```python
from build123d import *

# Parameters (mm, degrees)
BOSS_EXTRUDE1_DEPTH = 31.75
SKETCH2_R           = 1.366728635
CUT_EXTRUDE1_DEPTH  = 4.175
SKETCH4_W           = 7.9375
SKETCH4_H           = 4.7625
CUT_EXTRUDE2_DEPTH  = 4.175


with BuildPart() as part:
    # Sketch1 → Boss-Extrude1 (new body)
    with BuildSketch(Plane.XY):
        Polygon((0, 0), (25.4, 0), (25.4, 3.175), (3.175, 3.175), (3.175, 38.1), (0, 38.1), align=None)
    extrude(amount=BOSS_EXTRUDE1_DEPTH)

    # Sketch2 → Cut-Extrude1 (cut, through all)
    with BuildSketch(Plane(origin=(3.175, 0, 0), x_dir=(0, 0, -1), z_dir=(1, 0, 0))):
        with Locations((-25.4, 28.575)):
            Circle(SKETCH2_R)
        with Locations((-6.35, 28.575)):
            Circle(SKETCH2_R)
        with Locations((-25.4, 9.525)):
            Circle(SKETCH2_R)
        with Locations((-6.35, 9.525)):
            Circle(SKETCH2_R)
    extrude(amount=-CUT_EXTRUDE1_DEPTH, mode=Mode.SUBTRACT)

    # Sketch4 → Cut-Extrude2 (cut, through all)
    with BuildSketch(Plane(origin=(0, 3.175, 0), x_dir=(1, 0, 0), z_dir=(0, 1, 0))):
        with Locations((10.31875, -21.43125)):
            Rectangle(SKETCH4_W, SKETCH4_H)
        with Locations((10.31875, -10.31875)):
            Rectangle(SKETCH4_W, SKETCH4_H)
    extrude(amount=-CUT_EXTRUDE2_DEPTH, mode=Mode.SUBTRACT)


solid = part.part
```
Model file for the job. Use its own axes, mm. A direction names the side the tool comes from. Give positions to 0.01 mm unless a question says otherwise; leave off trailing zeros. Loops run counter-clockwise (first coordinate to the right, second up) from the corner with the lowest first, then second, coordinate; pieces in that order, holes last. Notation, with made-up numbers: (48, -21.75) -> (66, -21.75) arc R23 cw to (66, 4.25) -> close; hole circle Ø9 at (50.5, -24). An arc over 180 degrees is marked (long way). Use CSV: the item, a comma, the result in double quotes. Start each with the question number.
1) Flat gauge pins, fed straight in: pin 1 Ø5 at (x, z) = (21, 6) entering from +Y (3 decimals); pin 2 Ø1.5 at (x, y) = (5.5, 16.5) entering from -Z; pin 3 Ø8 at (y, z) = (29.5, 14.5) entering from +X (3 decimals). Where does each tip first touch, or does it go through?
2) Tool access for faces 4 (the flat face through (3.175, 20, 16)), 5 (the flat face through (14.288, 2, 21)), 6 (the cylindrical face through (1.61, 8.31, 5.72)): list every direction of +Z, -Z, +X, -X, +Y, -Y with a clear straight run to the whole face (end or side of a thin tool).
3) Slice it at C-C on x = 13.5. Give the number of separate pieces and of enclosed holes in the cut face, plus the area to 3 significant figures.
4) Slice it at B-B on z = 25.4. Give the cut face in (x, y) (3 decimals).
5) Mould opens along Y. For faces 1 (the cylindrical face through (1.6, 29, 24.1)), 2 (the flat face through (14, 3.175, 16)), 3 (the flat face through (0, 19, 16)) say: released by +Y, released by -Y, zero draft, split by the parting line, or undercut.
6) Slice it at D-D on y = 28. Give the cut face in (x, z) (3 decimals), plus the area to 3 significant figures.
7) Wall check: line 1 (Y direction, x = 1.35, z = 6.35); line 2 (Y direction, x = 16.25, z = 24) (3 decimals). Give the ranges that are in metal, low to high.
Computed values:
1,pin 1,"stops at y = 3.175"
1,pin 2,"passes through"
1,pin 3,"stops at x = 3.175"
2,face 4,"+Z, -Z, +X, +Y"
2,face 5,"+Y, -Y"
2,face 6,"+X, -X"
3,separate pieces,"3"
3,enclosed holes,"0"
3,area,"70.6 mm^2"
4,outline,"(0, 0) -> (25.4, 0) -> (25.4, 3.175) -> (3.175, 3.175) -> (3.175, 8.158) -> (0, 8.158) -> close; (0, 10.892) -> (3.175, 10.892) -> (3.175, 27.208) -> (0, 27.208) -> close; (0, 29.942) -> (3.175, 29.942) -> (3.175, 38.1) -> (0, 38.1) -> close"
5,face 1,"undercut"
5,face 2,"released by +Y"
5,face 3,"zero draft"
6,outline,"(0, 0) -> (3.175, 0) -> (3.175, 5.11) -> (0, 5.11) -> close; (0, 7.59) -> (3.175, 7.59) -> (3.175, 24.16) -> (0, 24.16) -> close; (0, 26.64) -> (3.175, 26.64) -> (3.175, 31.75) -> (0, 31.75) -> close"
6,area,"85.1 mm^2"
7,line 1,"y = 0 to 8.16, 10.89 to 27.21, 29.94 to 38.1"
7,line 2,"y = 0 to 3.175"
